from build123d import *

# Parameters (mm, degrees)
SKETCH_1_W          = 5
SKETCH_1_H          = 7.6
EXTRUDE_1_DEPTH     = 6.5
SKETCH_2_W          = 1
SKETCH_2_H          = 3.75
CUT_EXTRUDE_1_DEPTH = 2
SKETCH_3_W          = 4
SKETCH_3_H          = 4.87
CUT_EXTRUDE_2_DEPTH = 6.8
SKETCH_4_W          = 5
SKETCH_4_H          = 7.6
EXTRUDE_2_DEPTH     = 3.3
CHAMFER_1_SIZE      = 3.3
CHAMFER_1_SIZE2     = 1
CHAMFER_2_SIZE      = 3.3
CHAMFER_2_SIZE2     = 1.65
SKETCH_5_R          = 0.4
CUT_EXTRUDE_3_DEPTH = 5
SKETCH_6_R          = 1.75
CUT_EXTRUDE_4_DEPTH = 4.13


with BuildPart() as part:
    # Эскиз1 → Бобышка-Вытянуть1 (new body)
    with BuildSketch(Plane(origin=(0, 0, 0), x_dir=(1, 0, 0), z_dir=(0, 1, 0))):
        Rectangle(SKETCH_1_W, SKETCH_1_H)
    extrude(amount=EXTRUDE_1_DEPTH)

    # Эскиз2 → Вырез-Вытянуть1 (cut)
    with BuildSketch(Plane.XZ):
        with Locations((0, 1.925)):
            Rectangle(SKETCH_2_W, SKETCH_2_H)
    extrude(amount=-CUT_EXTRUDE_1_DEPTH, mode=Mode.SUBTRACT)

    # Эскиз3 → Вырез-Вытянуть2 (cut)
    with BuildSketch(Plane.XY.offset(3.8)):
        with Locations((0, 3.235)):
            Rectangle(SKETCH_3_W, SKETCH_3_H)
    extrude(amount=-CUT_EXTRUDE_2_DEPTH, mode=Mode.SUBTRACT)

    # Эскиз4 → Бобышка-Вытянуть2 (add)
    with BuildSketch(Plane(origin=(0, 6.5, 0), x_dir=(1, 0, 0), z_dir=(0, 1, 0))):
        Rectangle(SKETCH_4_W, SKETCH_4_H)
    extrude(amount=EXTRUDE_2_DEPTH)

    # Фаска1
    chamfer_1_edges = [part.edges().sort_by_distance(p)[0] for p in [
        (0, 9.8, 3.8),
    ]]
    chamfer_1_side = [part.faces().sort_by_distance(p)[0] for p in [
        (0, 6.154672702, 3.8),
    ]]
    chamfer(chamfer_1_edges, length=CHAMFER_1_SIZE, length2=CHAMFER_1_SIZE2, reference=chamfer_1_side[0])

    # Фаска2
    chamfer_2_edges = [part.edges().sort_by_distance(p)[0] for p in [
        (0, 9.8, -3.8),
    ]]
    chamfer_2_side = [part.faces().sort_by_distance(p)[0] for p in [
        (0, 4.9, -3.8),
    ]]
    chamfer(chamfer_2_edges, length=CHAMFER_2_SIZE, length2=CHAMFER_2_SIZE2, reference=chamfer_2_side[0])

    # Эскиз5 → Вырез-Вытянуть3 (cut)
    with BuildSketch(Plane.XZ.offset(-5.67)):
        with Locations(Location((0, -2.6, 0), (0, 0, 270))):
            Circle(SKETCH_5_R)
    extrude(amount=-CUT_EXTRUDE_3_DEPTH, mode=Mode.SUBTRACT)

    # Эскиз6 → Вырез-Вытянуть4 (cut)
    with BuildSketch(Plane(origin=(0, 9.8, 0), x_dir=(1, 0, 0), z_dir=(0, 1, 0))):
        with Locations(Location((0, -0.35, 0), (0, 0, 270))):
            Circle(SKETCH_6_R)
    extrude(amount=-CUT_EXTRUDE_4_DEPTH, mode=Mode.SUBTRACT)


solid = part.part
Here's how the part is built. I have some questions about the finished solid (model axes, mm). A direction names the side the tool comes from. Give positions to 0.01 mm unless a question says otherwise; leave off trailing zeros. Order: outer loops, then holes, each group sorted by start corner. A loop starts at its lowest first (then second) coordinate and runs counter-clockwise, first axis right, second up. Notation, with made-up numbers: (81.5, -10) -> (116.5, -10) arc R25 ccw to (116.5, 26) -> close; hole circle Ø8 at (-24.75, -24). An arc over 180 degrees is marked (long way). Use a Markdown table: item, result. Add a question column.
Item 1: Will these pins go through, and if not, where does the flat tip stop? pin 1 (1.2 mm diameter, centred on x = 1, y = 4, fed in from +Z); pin 2 (0.6 mm diameter, centred on x = 0, y = 0.5, fed in from +Z).
Item 2: Imagine slicing it at C-C on y = 8.5. Please give me the cut outline in (x, z), plus the area to 3 significant figures.
Item 3: For faces 1 (the face through (2, 3, 0)), 2 (the face through (-2, 9.8, 0)), 3 (the face through (-1.06, 7.76, -1.04)), which set-ups out of +Z, -Z, +X, -X, +Y, -Y let a thin tool reach every point of the face, with its end or its side?
Item 4: I need wall thicknesses on line 1 (Y direction, x = 1.8, z = 1.5); line 2 (X direction, y = 8.2, z = -2.6); line 3 (X direction, y = 5.25, z = 2). Which ranges of each line are inside material? Lowest first, please.
Item 5: If we mould it in two halves opening along X, with no side actions, what happens to faces 4 (the face through (0, 0.8, -0.3)), 5 (the face through (-1, 5.67, 2)), 6 (the face through (-2.5, 5, 0)), 7 (the face through (0, 0, -0.1))? For each: pulls with the +X half, pulls with the -X half, needs draft (parallel to the pull), parting line crosses it, or undercut.
Item 6: Imagine slicing it at B-B on y = 1.5. Please give me the cut outline in (x, z).
Item 7: Imagine slicing it at D-D on z = -1.75. Please give me the cut outline in (x, y).
Item 8: Imagine slicing it at A-A on z = 0.35. Please give me the cut outline in (x, y).
Data:
| question | item | result |
|---|---|---|
| 1 | pin 1 | stops at z = -3 |
| 1 | pin 2 | stops at z = 0.05 |
| 2 | outline | (-2.5, -2.8) -> (-0.35, -2.8) arc R0.4 cw (long way) to (0.35, -2.8) -> (2.5, -2.8) -> (2.5, 3.19) -> (-2.5, 3.19) -> close; hole circle Ø3.5 at (0, 0.35) |
| 2 | area | 19.9 mm² |
| 3 | face 1 | +Z |
| 3 | face 2 | +Z, -Z, +X, -X, +Y |
| 3 | face 3 | +Y |
| 4 | line 1 | y = 0 to 0.8, 5.67 to 9.8 |
| 4 | line 2 | x = -2.5 to -0.4, 0.4 to 2.5 |
| 4 | line 3 | x = -2.5 to -2, 2 to 2.5 |
| 5 | face 4 | undercut |
| 5 | face 5 | undercut |
| 5 | face 6 | pulls with the -X half |
| 5 | face 7 | needs draft |
| 6 | outline | (-2.5, -3.8) -> (2.5, -3.8) -> (2.5, 3.8) -> (2, 3.8) -> (2, -3) -> (-2, -3) -> (-2, 3.8) -> (-2.5, 3.8) -> close |
| 7 | outline | (-2.5, 0) -> (2.5, 0) -> (2.5, 9.8) -> (-2.5, 9.8) -> close; hole (-2, 0.8) -> (2, 0.8) -> (2, 5.67) -> (-2, 5.67) -> close |
| 8 | outline | (-2.5, 0) -> (-0.5, 0) -> (-0.5, 0.8) -> (-2, 0.8) -> (-2, 5.67) -> (-1.75, 5.67) -> (-1.75, 9.8) -> (-2.5, 9.8) -> close; (0.5, 0) -> (2.5, 0) -> (2.5, 9.8) -> (1.75, 9.8) -> (1.75, 5.67) -> (2, 5.67) -> (2, 0.8) -> (0.5, 0.8) -> close |
